Geometry: final body of the model. Coordinates: model frame, mm. Face numbers are marked on the shaded views. A direction names the side the tool comes from. Give positions to 0.01 mm unless a question says otherwise; leave off trailing zeros. Order: outer loops, then holes, each group sorted by start corner. A loop starts at its lowest first (then second) coordinate and runs counter-clockwise, first axis right, second up. Notation, with made-up numbers: (-26.75, 62) - (-0.75, 62) arc R15 ccw to (-0.75, 87) - close; hole circle Ø9 at (66, 7.25). An arc over 180 degrees is marked (long way). Put each result on its own line as item: value. Start each with the question number.
1. Section C-C on x = 19. Return the cut outline in (y, z) (3 decimals).
2. Set-up query: the marked faces 1 and 2. Return all of +Z, -Z, +X, -X, +Y, -Y with unobstructed straight access to the full face (end or side cutting, diameter ignored); none if empty.
3. Section D-D on y = 0. Return the cut outline in (x, z) (3 decimals).
4. First-contact query: P1, Ø10, axis at y = -9, z = -3.5, coming from the -X side. Flat tip, straight axial feed; report the tip coordinate or a pass-through.
5. Ray query, line 1 along Y through (x, z) = (0, 8.5); line 2 along Y through (x, z) = (-10, 5.5) (3 decimals); line 3 along Z through (x, y) = (9, 6.5) (3 decimals). Return the intervals inside material, ascending. Write a range as from..to.
6. Section A-A on z = -5.5. Return the cut outline in (x, y) (3 decimals), plus the area to 4 significant figures.
7. Section B-B on y = -12.5. Return the cut outline in (x, z) (3 decimals), plus the area to 4 significant figures.
8. Mould query, pull axis Z, two halves, no side actions, for the marked faces 3, 4 and 5. Classes: pulls with the +Z half, pulls with the -Z half, needs draft (parallel to the pull), parting line crosses it, or undercut.
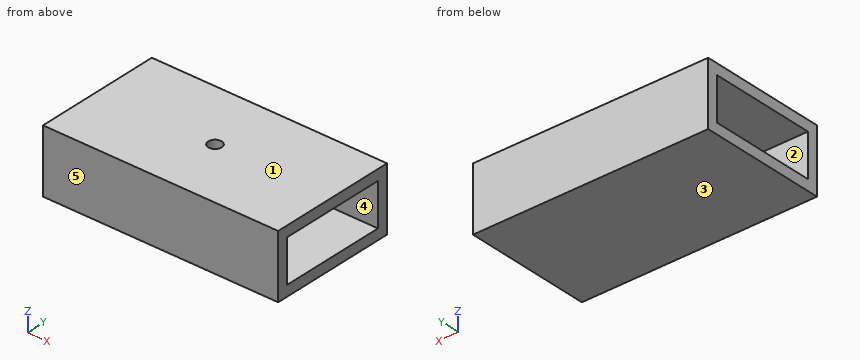
Autodesk Inventor part; units mm, degrees
ref_plane "YZ Plane" through (0, 0, 0) normal (1, 0, 0) x (0, 1, 0)
ref_plane "XZ Plane" through (0, 0, 0) normal (0, 1, 0) x (-1, 0, 0)
ref_plane "XY Plane" through (0, 0, 0) normal (0, 0, 1) x (1, 0, 0)
sketch "Sketch1" plane through (0, 0, 0) normal (1, 0, 0) x (0, 1, 0)
  line L0 (-15.875, -6.35) -> (15.875, -6.35)
  line L1 (15.875, -6.35) -> (15.875, 6.35)
  line L2 (15.875, 6.35) -> (-15.875, 6.35)
  line L3 (-15.875, 6.35) -> (-15.875, -6.35)
  line L4 (-15.875, -6.35) -> (15.875, 6.35) construction
  line L5 (15.875, -6.35) -> (-15.875, 6.35) construction
  line L6 (-19.05, -9.525) -> (19.05, -9.525)
  line L7 (19.05, -9.525) -> (19.05, 9.525)
  line L8 (19.05, 9.525) -> (-19.05, 9.525)
  line L9 (-19.05, 9.525) -> (-19.05, -9.525)
  line L10 (-19.05, -9.525) -> (19.05, 9.525) construction
  line L11 (19.05, -9.525) -> (-19.05, 9.525) construction
  point P0 (0, 0)
  dimension "d0" = 38.1
  dimension "d1" = 19.05
  dimension "d2" = 3.175
  dimension "d3" = 3.175
extrude "Extrusion1" add sketch "Sketch1" along normal mid plane 70
sketch "Sketch2" plane through (-35, -19.05, 9.525) normal (0, 0, 1) x (1, 0, 0)
  circle A0 centre (35, 19.05) radius 2
  dimension "d6" = 4
extrude "Extrusion2" cut sketch "Sketch2" against normal blind 10
equation "\"d3\" = d2"
properties part number "AluminumBlock"
Resolved:
1. outline: (-19.05, -9.525) - (19.05, -9.525) - (19.05, 9.525) - (-19.05, 9.525) - close; hole (-15.875, -6.35) - (15.875, -6.35) - (15.875, 6.35) - (-15.875, 6.35) - close
2. face 1: +Z, +X, -X, +Y, -Y
2. face 2: +X, -X
3. outline: (-35, -9.525) - (35, -9.525) - (35, -6.35) - (-35, -6.35) - close; (-35, 6.35) - (-2, 6.35) - (-2, 9.525) - (-35, 9.525) - close; (2, 6.35) - (35, 6.35) - (35, 9.525) - (2, 9.525) - close
4. P1: x = -35
5. line 1: -19.05..-2, 2..19.05
5. line 2: -19.05..-15.875, 15.875..19.05
5. line 3: -9.525..-6.35, 6.35..9.525
6. outline: (-35, -19.05) - (35, -19.05) - (35, -15.875) - (-35, -15.875) - close; (-35, 15.875) - (35, 15.875) - (35, 19.05) - (-35, 19.05) - close
6. area: 444.5 mm^2
7. outline: (-35, -9.525) - (35, -9.525) - (35, -6.35) - (-35, -6.35) - close; (-35, 6.35) - (35, 6.35) - (35, 9.525) - (-35, 9.525) - close
7. area: 444.5 mm^2
8. face 3: pulls with the -Z half
8. face 4: undercut
8. face 5: needs draft
